Geometry: final body of the model. Coordinates: model frame, mm. Face numbers are marked on the shaded views. A direction names the side the tool comes from. Coordinates: 2 decimals unless noted, no trailing zeros. Write each loop counter-clockwise with the first axis right and the second up, starting at its lowest first coordinate (ties: lowest second). Pieces come first, ordered by that corner, then holes. Notation, with made-up numbers: (87.25, -30) - (96.25, -30) arc R6 cw to (96.25, -25) - close; hole circle Ø7 at (-15, 61.25). An arc over 180 degrees is marked (long way). Put each result on its own line as item: value.
```python
from build123d import *

# Parameters (mm, degrees)
ESQUISSE1_R                                = 32.53
BOSS_EXTRU_1_DEPTH                         = 8.03
ESQUISSE2_R                                = 49.956
BOSS_EXTRU_2_DEPTH                         = 3.47
CHAMBRAGE_POUR_VIS_T_TE_HEXAGONALE_2_COUNT = 2
CHAMBRAGE_POUR_VIS_T_TE_HEXAGONALE_2_PITCH = 41.356
CHAMBRAGE_POUR_VIS_T_TE_HEXAGONALE_3_COUNT = 2
CHAMBRAGE_POUR_VIS_T_TE_HEXAGONALE_3_PITCH = 71.630693198
CHAMBRAGE_POUR_VIS_T_TE_HEXAGONALE_4_COUNT = 2
CHAMBRAGE_POUR_VIS_T_TE_HEXAGONALE_4_PITCH = 82.712
CHAMBRAGE_POUR_VIS_T_TE_HEXAGONALE_5_COUNT = 2
CHAMBRAGE_POUR_VIS_T_TE_HEXAGONALE_5_PITCH = 71.630693198
CHAMBRAGE_POUR_VIS_T_TE_HEXAGONALE_6_COUNT = 2
CHAMBRAGE_POUR_VIS_T_TE_HEXAGONALE_6_PITCH = 41.356


with BuildPart() as part:
    # Esquisse1 → Boss.-Extru.1 (new body)
    with BuildSketch(Plane(origin=(0, 0, 0), x_dir=(1, 0, 0), z_dir=(0, 1, 0))):
        Circle(ESQUISSE1_R)
    extrude(amount=-BOSS_EXTRU_1_DEPTH)

    # Esquisse2 → Boss.-Extru.2 (add)
    with BuildSketch(Plane(origin=(0, 0, 0), x_dir=(1, 0, 0), z_dir=(0, 1, 0))):
        Circle(ESQUISSE2_R)
    extrude(amount=BOSS_EXTRU_2_DEPTH)

    # Esquisse6 → Chambrage pour vis à tête hexagonale M33 (revolve, cut)
    with BuildSketch(Plane(origin=(-41.356, 3.47, 0), x_dir=(0, 0, 1), z_dir=(1, 0, 0))):
        Polygon((0, 0), (0, 11.5), (1.7, 11.5), (1.7, 2), (4.6755, 2), (4.6755, 0.025), (4.7005, 0), align=None)
    chambrage_pour_vis_t_te_hexagonale_m33 = revolve(axis=Axis((-41.356, 9.82, 0), (0, -1, 0)), mode=Mode.SUBTRACT)

    # Chambrage pour vis _ t_te hexagonale 2: Chambrage pour vis à tête hexagonale M33 ×2
    with Locations(*[Vector(0.5, 0, -0.866025404) * (i * CHAMBRAGE_POUR_VIS_T_TE_HEXAGONALE_2_PITCH) for i in range(1, CHAMBRAGE_POUR_VIS_T_TE_HEXAGONALE_2_COUNT)]):
        add(chambrage_pour_vis_t_te_hexagonale_m33, mode=Mode.SUBTRACT)

    # Chambrage pour vis _ t_te hexagonale 3: Chambrage pour vis à tête hexagonale M33 ×2
    with Locations(*[Vector(0.866025404, 0, -0.5) * (i * CHAMBRAGE_POUR_VIS_T_TE_HEXAGONALE_3_PITCH) for i in range(1, CHAMBRAGE_POUR_VIS_T_TE_HEXAGONALE_3_COUNT)]):
        add(chambrage_pour_vis_t_te_hexagonale_m33, mode=Mode.SUBTRACT)

    # Chambrage pour vis _ t_te hexagonale 4: Chambrage pour vis à tête hexagonale M33 ×2
    with Locations(*[(i * CHAMBRAGE_POUR_VIS_T_TE_HEXAGONALE_4_PITCH, 0, 0) for i in range(1, CHAMBRAGE_POUR_VIS_T_TE_HEXAGONALE_4_COUNT)]):
        add(chambrage_pour_vis_t_te_hexagonale_m33, mode=Mode.SUBTRACT)

    # Chambrage pour vis _ t_te hexagonale 5: Chambrage pour vis à tête hexagonale M33 ×2
    with Locations(*[Vector(0.866025404, 0, 0.5) * (i * CHAMBRAGE_POUR_VIS_T_TE_HEXAGONALE_5_PITCH) for i in range(1, CHAMBRAGE_POUR_VIS_T_TE_HEXAGONALE_5_COUNT)]):
        add(chambrage_pour_vis_t_te_hexagonale_m33, mode=Mode.SUBTRACT)

    # Chambrage pour vis _ t_te hexagonale 6: Chambrage pour vis à tête hexagonale M33 ×2
    with Locations(*[Vector(0.5, 0, 0.866025404) * (i * CHAMBRAGE_POUR_VIS_T_TE_HEXAGONALE_6_PITCH) for i in range(1, CHAMBRAGE_POUR_VIS_T_TE_HEXAGONALE_6_COUNT)]):
        add(chambrage_pour_vis_t_te_hexagonale_m33, mode=Mode.SUBTRACT)


solid = part.part
```
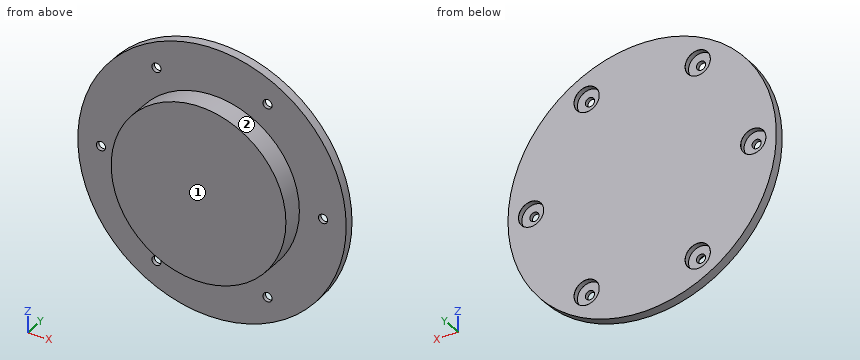
1. Section query A-A (z = 0). Count the separate pieces of the cut face and the enclosed holes in it, then the cut area to 3 significant figures.
Answer below:
separate pieces: 3
enclosed holes: 0
area: 822 mm²
2. Ray query, probe 1 along X at (y, z) = (2.05, 0); probe 2 along X at (y, z) = (0.9, 0); probe 3 along Y at (x, z) = (38, 22.5). Return the intervals inside material, ascending. Write a range as from..to.
Answer below:
probe 1: x = -49.96..-46.03, -36.68..36.68, 46.03..49.96
probe 2: x = -49.96..-43.06, -39.66..39.66, 43.06..49.96
probe 3: y = 0..3.47
3. Section query B-B (x = 0). Return loops of the section in (y, z), then the cut area to 3 significant figures.
Answer below:
outline: (-8.03, -32.53) - (0, -32.53) - (0, -49.96) - (3.47, -49.96) - (3.47, 49.96) - (0, 49.96) - (0, 32.53) - (-8.03, 32.53) - close
area: 869 mm²
4. Section query D-D (z = -10). Return loops of the section in (x, y), then the cut area to 3 significant figures.
Answer below:
outline: (-48.94, 0) - (-30.95, 0) - (-30.95, -8.03) - (30.95, -8.03) - (30.95, 0) - (48.94, 0) - (48.94, 3.47) - (-48.94, 3.47) - close
area: 837 mm²
5. Set-up query: the marked faces 1 and 2. Return all of +Z, -Z, +X, -X, +Y, -Y with unobstructed straight access to the full face (end or side cutting, diameter ignored); none if empty.
Answer below:
face 1: +Z, -Z, +X, -X, -Y
face 2: -Y
6. Section query C-C (y = -2). Return loops of the section in (x, z).
Answer below:
outline: circle Ø65.06 at (0, 0)
7. Pin query (flat end, axial travel): pin 1 Ø3 at (x, y) = (3.5, 1.5) entering from +Z; pin 2 Ø5.5 at (x, z) = (-41.356, 0) entering from -Y; pin 3 Ø7.5 at (x, z) = (20.68, -35.82) entering from +Y. Return the tip coordinate at first contact, or that it passes through.
Answer below:
pin 1: stops at z = 49.92
pin 2: stops at y = 0
pin 3: stops at y = 1.47
